For this review, use the dimensioned drawing (mm, ordinates from the lowest corner) and the shaded views. Coordinates: 2 decimals unless noted, no trailing zeros. Loops run counter-clockwise (first coordinate to the right, second up) from the corner with the lowest first, then second, coordinate; pieces in that order, holes last. Notation, with made-up numbers: M -1,69.5 L 12,69.5 A22 ccw 12,94.5 Z; hole C 58,81 d11. An arc over 180 degrees is marked long. Use CSV: the item, a comma, the result in double quotes. Start each with the question number.
1. Add section A-A, the plane z = 13. Write out the cut boundary in (x, y), then the cut area to 3 significant figures.
2. Add section B-B, the plane x = 61. Write out the cut boundary in (y, z).
3. For L1, parallel to Y at x = 40, z = 26 (1 decimal); L2, parallel to Y at x = 41, z = 21, list the stretches that pass through material, from the lowest coordinate up.
4. Clearance check with flat-ended pins moving along their axes: P1, Ø4, axis at x = 37.5, z = 48, coming from the +Y side (1 decimal); P2, Ø5, axis at x = 52.5, z = 16.5, coming from the -Y side; P3, Ø4, axis at x = 12, z = 55, coming from the +Y side. State where each tip first meets the part, or that it passes through.
5. Add section C-C, the plane y = 88. Write out the cut boundary in (x, z).
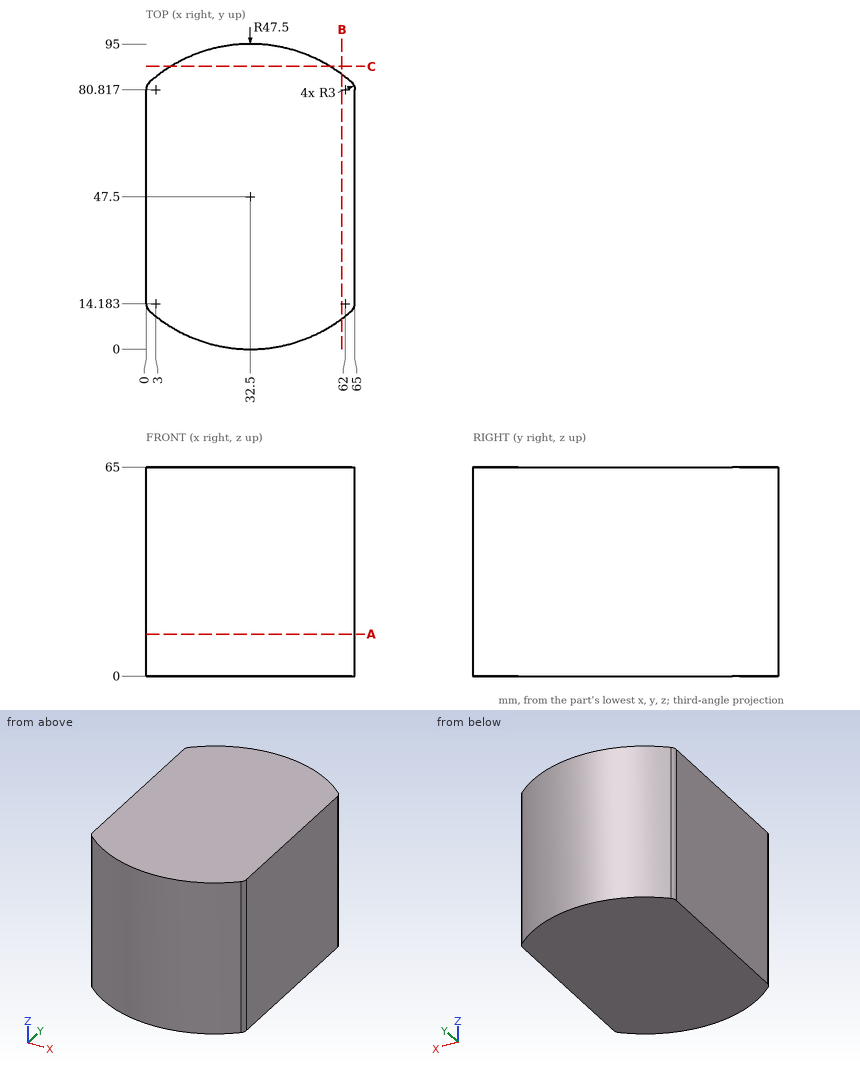
Computed:
1,outline,"M 0,14.18 A3 ccw 1.01,11.94 A47.5 ccw 63.99,11.94 A3 ccw 65,14.18 L 65,80.82 A3 ccw 63.99,83.06 A47.5 ccw 1.01,83.06 A3 ccw 0,80.82 Z"
1,area,"5,650 mm^2"
2,outline,"M 9.5,0 L 85.5,0 L 85.5,65 L 9.5,65 Z"
3,L1,"y = 0.6 to 94.4"
3,L2,"y = 0.77 to 94.23"
4,P1,"stops at y = 94.9"
4,P2,"stops at y = 3.34"
4,P3,"stops at y = 91.25"
5,outline,"M 7.68,0 L 57.32,0 L 57.32,65 L 7.68,65 Z"
